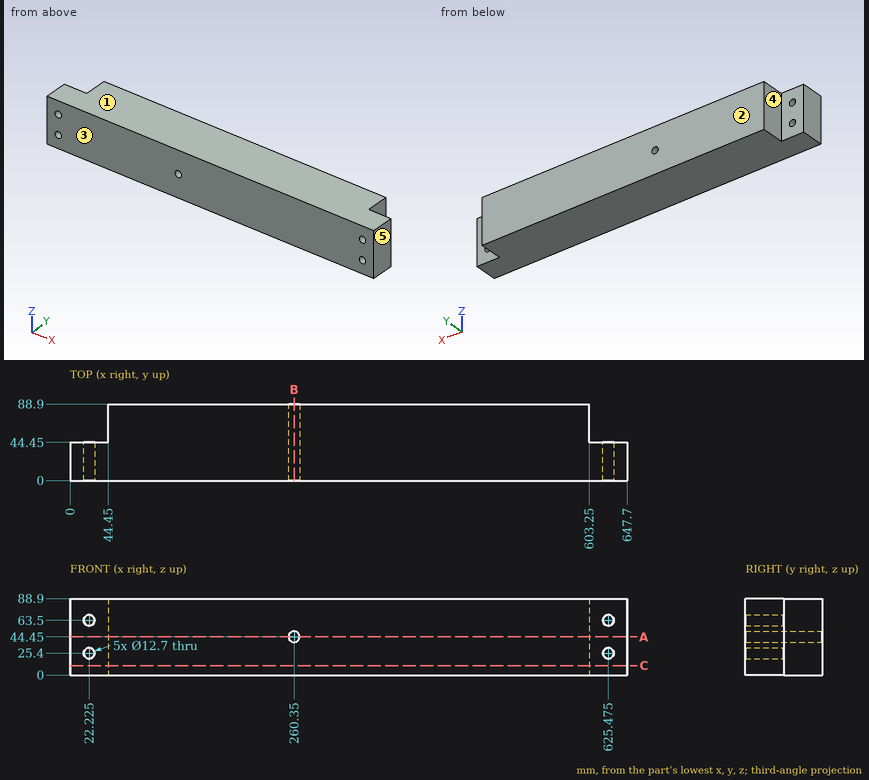
Check sheet for the drawn part. Datum: minimum x, y, z corner. Units: mm. A direction names the side the tool comes from. Round coordinates to 2 decimals unless told otherwise and drop trailing zeros. Order: outer loops, then holes, each group sorted by start corner. A loop starts at its lowest first (then second) coordinate and runs counter-clockwise, first axis right, second up. Notation, with made-up numbers: M 56.25,35 L 94.25,35 A12 cw 94.25,46 Z; hole C -2.5,-1 d6. An arc over 180 degrees is marked long. Answer in a Markdown table with one row per item.
(1) Gauge pin test, flat ends, axial feed: pin 1 (10 mm diameter, centred on x = 378.5, z = 52, fed in from -Y); pin 2 (14.5 mm diameter, centred on x = 22.225, z = 63.5, fed in from +Y); pin 3 (11.5 mm diameter, centred on x = 625.475, z = 63.5, fed in from -Y) (3 decimals); pin 4 (13.5 mm diameter, centred on y = 68, z = 55.5, fed in from -X). Record the tip position at first contact, or that the pin passes through.
Findings:
| item | result |
|---|---|
| pin 1 | stops at y = 0 |
| pin 2 | stops at y = 44.45 |
| pin 3 | passes through |
| pin 4 | stops at x = 44.45 |
(2) Material ranges on line 1 along X through (y, z) = (17, 63); line 2 along X through (y, z) = (32.5, 21); line 3 along Y through (x, z) = (39.5, 59), recorded low to high. Write a range as from..to.
Findings:
| item | result |
|---|---|
| line 1 | x = 0..15.89, 28.56..619.14, 631.81..647.7 |
| line 2 | x = 0..17.65, 26.8..620.9, 630.05..647.7 |
| line 3 | y = 0..44.45 |
(3) Draft check along Y on the marked faces 1, 2 and 3. Enter one of: +Y half, -Y half, draft (parallel to the pull), parting line (faces both ways), or undercut.
Findings:
| item | result |
|---|---|
| face 1 | draft |
| face 2 | +Y half |
| face 3 | -Y half |
(4) Section check C-C on z = 11. Record the boundary of the cut face in (x, y).
Findings:
| item | result |
|---|---|
| outline | M 0,0 L 647.7,0 L 647.7,44.45 L 603.25,44.45 L 603.25,88.9 L 44.45,88.9 L 44.45,44.45 L 0,44.45 Z |
(5) Set-up check for the marked faces 4 and 5: record each of +Z, -Z, +X, -X, +Y, -Y from which the full face is reachable in a straight line by a thin tool's end or side.
Findings:
| item | result |
|---|---|
| face 4 | +Z, -Z, -X, +Y |
| face 5 | +Z, -Z, +X, +Y, -Y |
(6) Section check A-A on z = 44.45. Record the boundary of the cut face in (x, y), plus the area to 3 significant figures.
Findings:
| item | result |
|---|---|
| outline | M 0,0 L 254,0 L 254,88.9 L 44.45,88.9 L 44.45,44.45 L 0,44.45 Z; M 266.7,0 L 647.7,0 L 647.7,44.45 L 603.25,44.45 L 603.25,88.9 L 266.7,88.9 Z |
| area | 52,500 mm^2 |
(7) Section check B-B on x = 260.35. Record the boundary of the cut face in (y, z), plus the area to 3 significant figures.
Findings:
| item | result |
|---|---|
| outline | M 0,0 L 88.9,0 L 88.9,38.1 L 0,38.1 Z; M 0,50.8 L 88.9,50.8 L 88.9,88.9 L 0,88.9 Z |
| area | 6,770 mm^2 |
